Part model, mm, in its own coordinate system. Face numbers are marked on the shaded views. A direction names the side the tool comes from. Round coordinates to 2 decimals unless told otherwise and drop trailing zeros. Write each loop counter-clockwise with the first axis right and the second up, starting at its lowest first coordinate (ties: lowest second). Pieces come first, ordered by that corner, then holes. Notation, with made-up numbers: M -37,5 L -20,5 A28 cw -20,43 Z; hole C -28.75,-2 d5. An arc over 180 degrees is marked long. Use one line per item in the form item = value. Start each with the question number.
Item 1: Cut at C-C, the plane z = 23.5. State how many separate pieces and enclosed holes the cut face has, then the cut area to 3 significant figures.
Item 2: Which spindle directions (+Z, -Z, +X, -X, +Y, -Y) get a long thin tool onto all of the face, cutting with end or side? Do the marked faces 1, 2, 3 and 4. Say none if no direction does.
Item 3: Flat gauge pins, fed straight in: pin 1 Ø5.5 at (x, y) = (-85.65, -19.98) entering from -Z; pin 2 Ø1.8 at (x, z) = (-6, 22.5) entering from -Y; pin 3 Ø10 at (y, z) = (-5, 13.5) entering from +X; pin 4 Ø6.5 at (y, z) = (-15, 9.5) entering from +X. Where does each tip first touch, or does it go through?
Item 4: Probe L1, parallel to X at y = 20.8, z = 15.5; L2, parallel to Y at x = -80, z = 26; L3, parallel to X at y = -19.35, z = 10.5. List the from-to ranges inside material, lowest first.
Item 5: Cut at A-A, the plane z = 5.5. Give the cut face in (x, y).
Item 6: Cut at B-B, the plane z = 15.5. Give the cut face in (x, y), then the cut area to 3 significant figures.
from build123d import *

# Parameters (mm, degrees)
SKETCH1_W             = 10
SKETCH1_H             = 5
BOSS_EXTRUDE1_DEPTH   = 21
BOSS_EXTRUDE1_2_DEPTH = 21
BOSS_EXTRUDE2_DEPTH   = 6
SKETCH3_W             = 20.5
SKETCH3_H             = 5
BOSS_EXTRUDE3_DEPTH   = 21
CUT_EXTRUDE1_REACH    = 64.414
SKETCH4_R             = 1.65
CUT_EXTRUDE2_REACH    = 61.08
SKETCH5_R             = 2.2
SKETCH6_R             = 1.75
BOSS_EXTRUDE4_DEPTH   = 6
CUT_EXTRUDE3_REACH    = 107.857
CUT_EXTRUDE7_REACH    = 109.208
BOSS_EXTRUDE5_DEPTH   = 6
BOSS_EXTRUDE6_DEPTH   = 3
BOSS_EXTRUDE7_DEPTH   = 3
BOSS_EXTRUDE8_DEPTH   = 20.5
CUT_EXTRUDE9_DEPTH    = 6
FILLET1_R             = 1
CUT_EXTRUDE10_DEPTH   = 2


with BuildPart() as part:
    # Sketch1 → Boss-Extrude1 (new body)
    with BuildSketch(Plane.XY):
        with Locations((-31.296703297, 19.79010989)):
            Rectangle(SKETCH1_W, SKETCH1_H)
    extrude(amount=BOSS_EXTRUDE1_DEPTH)



with BuildPart() as body_2:
    # Sketch1 → Boss-Extrude1 2 (new body)
    with BuildSketch(Plane.XY):
        with Locations((19.703296703, 19.79010989)):
            Rectangle(SKETCH1_W, SKETCH1_H)
    extrude(amount=BOSS_EXTRUDE1_2_DEPTH)


with BuildPart() as part_1:
    add(part.part)

    add(body_2.part)  # Boss-Extrude2 merges body 2
    # Sketch2 → Boss-Extrude2 (add)
    with BuildSketch(Plane.XY.offset(21)):
        Polygon((-36.296703297, 22.29010989), (24.703296703, 22.29010989), (24.703296703, 7.29010989), (12.703296703, 7.29010989), (-5.796703297, -11.20989011), (-5.796703297, -20.70989011), (-36.296703297, -20.70989011), align=None)
    extrude(amount=BOSS_EXTRUDE2_DEPTH)

    # Sketch3 → Boss-Extrude3 (add)
    with BuildSketch(Plane(origin=(0, 0, 21), x_dir=(-1, 0, 0), z_dir=(0, 0, -1))):
        with Locations((16.046703297, -18.20989011)):
            Rectangle(SKETCH3_W, SKETCH3_H)
    extrude(amount=BOSS_EXTRUDE3_DEPTH)

    # Sketch4 → Cut-Extrude1 (cut, up to next)
    with BuildSketch(Plane(origin=(0, 22.29010989, 0), x_dir=(1, 0, 0), z_dir=(0, 1, 0)), mode=Mode.PRIVATE) as cut_extrude1_sk1:
        with Locations(Location((-29.796703297, -5.5, 0), (0, 0, 270))):
            Circle(SKETCH4_R)
    cut_extrude1_tool1 = extrude(cut_extrude1_sk1.sketch, amount=-CUT_EXTRUDE1_REACH, mode=Mode.PRIVATE) & part_1.part
    # Sketch4 → Cut-Extrude1 (cut, up to next)
    with BuildSketch(Plane(origin=(0, 22.29010989, 0), x_dir=(1, 0, 0), z_dir=(0, 1, 0)), mode=Mode.PRIVATE) as cut_extrude1_sk2:
        with Locations(Location((18.203296703, -5.5, 0), (0, 0, 270))):
            Circle(SKETCH4_R)
    cut_extrude1_tool2 = extrude(cut_extrude1_sk2.sketch, amount=-CUT_EXTRUDE1_REACH, mode=Mode.PRIVATE) & part_1.part
    # Sketch4 → Cut-Extrude1 (cut, up to next)
    with BuildSketch(Plane(origin=(0, 22.29010989, 0), x_dir=(1, 0, 0), z_dir=(0, 1, 0)), mode=Mode.PRIVATE) as cut_extrude1_sk3:
        with Locations(Location((18.203296703, -15.5, 0), (0, 0, 270))):
            Circle(SKETCH4_R)
    cut_extrude1_tool3 = extrude(cut_extrude1_sk3.sketch, amount=-CUT_EXTRUDE1_REACH, mode=Mode.PRIVATE) & part_1.part
    # Sketch4 → Cut-Extrude1 (cut, up to next)
    with BuildSketch(Plane(origin=(0, 22.29010989, 0), x_dir=(1, 0, 0), z_dir=(0, 1, 0)), mode=Mode.PRIVATE) as cut_extrude1_sk4:
        with Locations(Location((-29.796703297, -15.5, 0), (0, 0, 270))):
            Circle(SKETCH4_R)
    cut_extrude1_tool4 = extrude(cut_extrude1_sk4.sketch, amount=-CUT_EXTRUDE1_REACH, mode=Mode.PRIVATE) & part_1.part
    add(cut_extrude1_tool1.solids().sort_by_distance((-29.796703, 22.29011, 5.5))[0], mode=Mode.SUBTRACT)
    add(cut_extrude1_tool2.solids().sort_by_distance((18.203297, 22.29011, 5.5))[0], mode=Mode.SUBTRACT)
    add(cut_extrude1_tool3.solids().sort_by_distance((18.203297, 22.29011, 15.5))[0], mode=Mode.SUBTRACT)
    add(cut_extrude1_tool4.solids().sort_by_distance((-29.796703, 22.29011, 15.5))[0], mode=Mode.SUBTRACT)

    # Sketch5 → Cut-Extrude2 (cut, up to next)
    with BuildSketch(Plane(origin=(0, -15.70989011, 0), x_dir=(1, 0, 0), z_dir=(0, 1, 0)), mode=Mode.PRIVATE) as cut_extrude2_sk1:
        with Locations(Location((-16.046703297, -10.5, 0), (0, 0, 270))):
            Circle(SKETCH5_R)
    cut_extrude2_tool1 = extrude(cut_extrude2_sk1.sketch, amount=-CUT_EXTRUDE2_REACH, mode=Mode.PRIVATE) & part_1.part
    add(cut_extrude2_tool1.solids().sort_by_distance((-16.046703, -15.70989, 10.5))[0], mode=Mode.SUBTRACT)

    # Sketch6 → Boss-Extrude4 (add)
    with BuildSketch(Plane.XY.offset(27)):
        with BuildLine():
            Line((-79.859138265, -39.735236509), (-51.503727763, -19.880564327))
            add(Edge.make_bspline(
                [(-51.503727763, -19.880564327), (-43.777944292, -18.491061957), (-36.296703297, -20.70989011)],
                knots=[0, 0, 0, 1, 1, 1], degree=2))
            Line((-36.296703297, -20.70989011), (-36.296703297, 22.29010989))
            add(Edge.make_bspline(
                [(-57.962836939, 19.661219133), (-46.447122218, 13.814864777), (-36.296703297, 22.29010989)],
                knots=[0, 0, 0, 1, 1, 1], degree=2))
            add(Edge.make_bspline(
                [(-95.842115451, -15.524174544), (-74.909238175, -0.080881368), (-57.962836939, 19.661219133)],
                knots=[0, 0, 0, 1, 1, 1], degree=2))
            add(Edge.make_bspline(
                [(-95.842115451, -15.524174544), (-85.086697095, -25.754599345), (-79.859138265, -39.735236509)],
                knots=[0, 0, 0, 1, 1, 1], degree=2))
        make_face()
        with Locations((-40.590214383, -0.641481396)):
            Circle(SKETCH6_R, mode=Mode.SUBTRACT)
        with Locations((-85.645276872, -19.981629898)):
            Circle(SKETCH6_R, mode=Mode.SUBTRACT)
        with Locations((-79.909512508, -28.173150341)):
            Circle(SKETCH6_R, mode=Mode.SUBTRACT)
        with Locations((-46.325978746, 7.550039047)):
            Circle(SKETCH6_R, mode=Mode.SUBTRACT)
        Polygon((-85.932915117, -13.468776127), (-52.347681301, 10.047857763), (-40.302576138, -7.154335167), (-73.887809953, -30.670969058), align=None, mode=Mode.SUBTRACT)
    extrude(amount=-BOSS_EXTRUDE4_DEPTH)

    # Sketch7 → Cut-Extrude3 (cut, up to next)
    with BuildSketch(Plane(origin=(0, 0, 21), x_dir=(-1, 0, 0), z_dir=(0, 0, -1)), mode=Mode.PRIVATE) as cut_extrude3_sk1:
        with BuildLine():
            Line((36.296703297, -20.70989011), (26.296703297, -20.70989011))
            add(Edge.make_bspline(
                [(26.296703297, -20.70989011), (39.15974316, -13.056772406), (51.503727763, -19.880564327)],
                knots=[0, 0, 0, 1, 1, 1], degree=2))
            add(Edge.make_bspline(
                [(51.503727763, -19.880564327), (43.777944292, -18.491061957), (36.296703297, -20.70989011)],
                knots=[0, 0, 0, 1, 1, 1], degree=2))
        make_face()
    cut_extrude3_tool1 = extrude(cut_extrude3_sk1.sketch, amount=-CUT_EXTRUDE3_REACH, mode=Mode.PRIVATE) & part_1.part
    add(cut_extrude3_tool1.solids().sort_by_distance((-38.072503, -18.786508, 21))[0], mode=Mode.SUBTRACT)

    # Sketch10 → Cut-Extrude7 (cut, up to next)
    with BuildSketch(Plane.XY.offset(27), mode=Mode.PRIVATE) as cut_extrude7_sk1:
        with BuildLine():
            Line((5.266834936, 14.29010989), (-27.788194587, 14.29010989))
            add(Edge.make_bspline(
                [(-27.788194587, 14.29010989), (-23.431396766, 3.132914333), (-25.823714091, -8.70989011)],
                knots=[0, 0, 0, 1, 1, 1], degree=2))
            Line((-25.823714091, -8.70989011), (-13.796703297, -8.70989011))
            add(Edge.make_bspline(
                [(5.266834936, 14.29010989), (-9.842167425, 7.185288479), (-13.796703297, -8.70989011)],
                knots=[0, 0, 0, 1, 1, 1], degree=2))
        make_face()
    cut_extrude7_tool1 = extrude(cut_extrude7_sk1.sketch, amount=-CUT_EXTRUDE7_REACH, mode=Mode.PRIVATE) & part_1.part
    add(cut_extrude7_tool1.solids().sort_by_distance((-15.764918, 4.836925, 27))[0], mode=Mode.SUBTRACT)

    # Sketch11 → Boss-Extrude5 (add)
    with BuildSketch(Plane.XY.offset(27)):
        with BuildLine():
            Line((15.119169314, 7.29010989), (12.703296703, 7.29010989))
            Line((12.703296703, 7.29010989), (-5.796703297, -11.20989011))
            Line((-5.796703297, -11.20989011), (-5.796703297, -20.70989011))
            add(Edge.make_bspline(
                [(-5.796703297, -20.70989011), (-0.06692684, -3.022661062), (15.119169314, 7.29010989)],
                knots=[0, 0, 0, 1, 1, 1], degree=2))
        make_face()
    extrude(amount=-BOSS_EXTRUDE5_DEPTH)

    # Sketch12 → Boss-Extrude6 (add)
    with BuildSketch(Plane(origin=(24.703296703, 0, 0), x_dir=(0, 0, -1), z_dir=(1, 0, 0))):
        Polygon((-21, 11.29010989), (-9, 17.29010989), (-21, 17.29010989), align=None)
    extrude(amount=-BOSS_EXTRUDE6_DEPTH)

    # Sketch13 → Boss-Extrude7 (add)
    with BuildSketch(Plane.ZY.offset(36.296703297)):
        Polygon((21, 11.29010989), (21, 17.29010989), (9, 17.29010989), align=None)
    extrude(amount=-BOSS_EXTRUDE7_DEPTH)

    # Sketch14 → Boss-Extrude8 (add)
    with BuildSketch(Plane(origin=(-5.796703297, 0, 0), x_dir=(0, 0, -1), z_dir=(1, 0, 0))):
        Polygon((-17.7, -15.70989011), (-21, -12.40989011), (-21, -15.70989011), align=None)
    extrude(amount=-BOSS_EXTRUDE8_DEPTH)

    # Sketch15 → Cut-Extrude9 (cut)
    with BuildSketch(Plane.XY.offset(27)):
        with BuildLine():
            Line((24.703296703, 7.29010989), (24.703296703, 11.09010989))
            add(Edge.make_bspline(
                [(-5.796703297, -20.70989011), (1.890928929, 9.845343686), (24.703296703, 11.09010989)],
                knots=[0, 0, 0, 1, 1, 1], degree=2))
            add(Edge.make_bspline(
                [(-5.796703297, -20.70989011), (-0.06692684, -3.022661062), (15.119169314, 7.29010989)],
                knots=[0, 0, 0, 1, 1, 1], degree=2))
            Line((15.119169314, 7.29010989), (24.703296703, 7.29010989))
        make_face()
    extrude(amount=-CUT_EXTRUDE9_DEPTH, mode=Mode.SUBTRACT)

    # Fillet1
    fillet1_edges = [part_1.edges().sort_by_distance(p)[0] for p in [
        (-95.842115451, -15.524174544, 24),
        (-57.962836939, 19.661219133, 24),
        (-79.859138265, -39.735236509, 24),
    ]]
    fillet(fillet1_edges, radius=FILLET1_R)

    # Sketch16 → Cut-Extrude10 (cut)
    with BuildSketch(Plane(origin=(0, -15.70989011, 0), x_dir=(1, 0, 0), z_dir=(0, 1, 0))):
        Polygon((-13.910507301, -6.8), (-18.182899293, -6.8), (-20.319095289, -10.5), (-18.182899293, -14.2), (-13.910507301, -14.2), (-11.774311305, -10.5), align=None)
    extrude(amount=-CUT_EXTRUDE10_DEPTH, mode=Mode.SUBTRACT)


solid = part_1.part
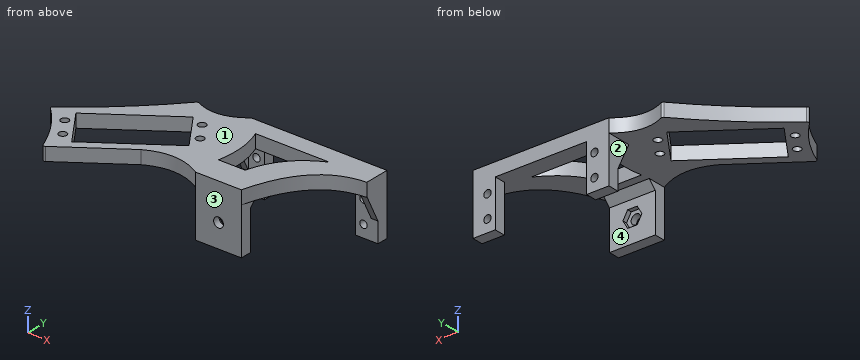
Model answer:
q1.separate_pieces = 1
q1.enclosed_holes = 6
q1.area = 2,520 mm²
q2.face_1 = +Z, +X, -X, +Y, -Y
q2.face_2 = -Z, -X, +Y, -Y
q2.face_3 = +Z, -Z, +X, -Y
q2.face_4 = -Z, +X, -X, +Y
q3.pin_1 = 21
q3.pin_2 = -20.71
q3.pin_3 = through
q3.pin_4 = -5.8
q4.L1 = -36.3 to -31.45, -28.15 to -26.3, 14.7 to 16.55, 19.85 to 24.7
q4.L2 = -38.97 to -29.92, -26.43 to -21.94, -9.31 to -2.72
q4.L3 = -26.3 to -18.25, -13.85 to -5.8
q5.outline = M -36.3,17.29 L -31.45,17.29 L -31.45,22.29 L -36.3,22.29 Z; M -28.15,17.29 L -26.3,17.29 L -26.3,22.29 L -28.15,22.29 Z; M -26.3,-20.71 L -5.8,-20.71 L -5.8,-15.71 L -26.3,-15.71 Z; M 14.7,17.29 L 16.55,17.29 L 16.55,22.29 L 14.7,22.29 Z; M 19.85,17.29 L 24.7,17.29 L 24.7,22.29 L 19.85,22.29 Z
q6.outline = M -36.3,14.04 L -33.3,14.04 L -33.3,17.29 L -31.45,17.29 L -31.45,22.29 L -36.3,22.29 Z; M -28.15,17.29 L -26.3,17.29 L -26.3,22.29 L -28.15,22.29 Z; M -26.3,-20.71 L -5.8,-20.71 L -5.8,-15.71 L -26.3,-15.71 Z; M 14.7,17.29 L 16.55,17.29 L 16.55,22.29 L 14.7,22.29 Z; M 19.85,17.29 L 21.7,17.29 L 21.7,14.04 L 24.7,14.04 L 24.7,22.29 L 19.85,22.29 Z
q6.area = 189 mm²
